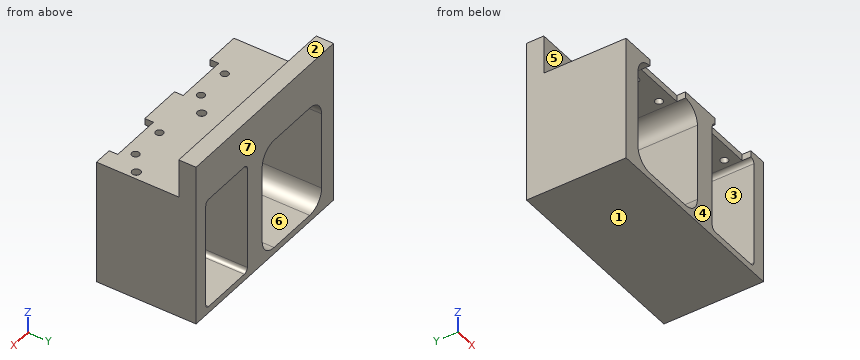
from build123d import *

# Parameters (mm, degrees)
SKETCH1_W                  = 405
SKETCH1_H                  = 295
BOSS_EXTRUDE1_DEPTH        = 53
SKETCH3_OUTSIDE_W          = 507.768
SKETCH3_OUTSIDE_H          = 397.768
SKETCH3_OUTSIDE_W_2        = 369
SKETCH3_OUTSIDE_H_2        = 259
CUT_EXTRUDE2_DEPTH         = 45
MINI_BIN_CUTS_DEPTH        = 46
FILLET1_R                  = 8
SKETCH6_W                  = 259
SKETCH6_H                  = 7
CUT_EXTRUDE5_DEPTH         = 418.533531588
SKETCH8_R                  = 1.75
SKETCH8_R_2                = 1.95
HOLES_LIDS_8_9_12_13_DEPTH = 3
SKETCH9_W                  = 113
SKETCH9_H                  = 46
SKETCH9_W_2                = 199.5
CUT_EXTRUDE6_DEPTH         = 362.718467872
SKETCH10_W                 = 219
SKETCH10_H                 = 46
CUT_EXTRUDE7_DEPTH         = 182.993131739
CUT_EXTRUDE8_REACH         = 121.093
SKETCH11_W                 = 24
SKETCH11_H                 = 4


with BuildPart() as part:
    # Sketch1 → Boss-Extrude1 (new body)
    with BuildSketch(Plane(origin=(0, 0, 0), x_dir=(1, 0, 0), z_dir=(0, 1, 0))):
        Rectangle(SKETCH1_W, SKETCH1_H)
    extrude(amount=BOSS_EXTRUDE1_DEPTH)

    # Sketch3 outside → Cut-Extrude2 (cut)
    with BuildSketch(Plane(origin=(0, 0, 0), x_dir=(-1, 0, 0), z_dir=(0, -1, 0))):
        Rectangle(SKETCH3_OUTSIDE_W, SKETCH3_OUTSIDE_H)
        Rectangle(SKETCH3_OUTSIDE_W_2, SKETCH3_OUTSIDE_H_2, mode=Mode.SUBTRACT)
    extrude(amount=-CUT_EXTRUDE2_DEPTH, mode=Mode.SUBTRACT)

    # Sketch2 → Mini bin cuts (cut)
    with BuildSketch(Plane(origin=(0, 53, 0), x_dir=(1, 0, 0), z_dir=(0, 1, 0))):
        with BuildLine():
            Line((-173.5, -126.5), (-105.5, -126.5))
            ThreePointArc((-105.5, -126.5), (-99.843145751, -124.156854249), (-97.5, -118.5))
            Line((-97.5, -118.5), (-97.5, -49.5))
            ThreePointArc((-97.5, -49.5), (-99.843145751, -43.843145751), (-105.5, -41.5))
            Line((-105.5, -41.5), (-173.5, -41.5))
            ThreePointArc((-173.5, -41.5), (-179.156854249, -43.843145751), (-181.5, -49.5))
            Line((-181.5, -49.5), (-181.5, -118.5))
            ThreePointArc((-181.5, -118.5), (-179.156854249, -124.156854249), (-173.5, -126.5))
        make_face()
        with BuildLine():
            Line((-173.5, -31.5), (-105.5, -31.5))
            ThreePointArc((-105.5, -31.5), (-99.843145751, -29.156854249), (-97.5, -23.5))
            Line((-97.5, -23.5), (-97.5, 40.5))
            ThreePointArc((-97.5, 40.5), (-99.843145751, 46.156854249), (-105.5, 48.5))
            Line((-105.5, 48.5), (-173.5, 48.5))
            ThreePointArc((-173.5, 48.5), (-179.156854249, 46.156854249), (-181.5, 40.5))
            Line((-181.5, 40.5), (-181.5, -23.5))
            ThreePointArc((-181.5, -23.5), (-179.156854249, -29.156854249), (-173.5, -31.5))
        make_face()
        with BuildLine():
            Line((-173.5, 126.5), (-105.5, 126.5))
            ThreePointArc((-105.5, 126.5), (-99.843145751, 124.156854249), (-97.5, 118.5))
            Line((-97.5, 118.5), (-97.5, 66.5))
            ThreePointArc((-97.5, 66.5), (-99.843145751, 60.843145751), (-105.5, 58.5))
            Line((-105.5, 58.5), (-173.5, 58.5))
            ThreePointArc((-173.5, 58.5), (-179.156854249, 60.843145751), (-181.5, 66.5))
            Line((-181.5, 66.5), (-181.5, 118.5))
            ThreePointArc((-181.5, 118.5), (-179.156854249, 124.156854249), (-173.5, 126.5))
        make_face()
        with BuildLine():
            Line((173.5, -126.5), (115.5, -126.5))
            ThreePointArc((115.5, -126.5), (109.843145751, -124.156854249), (107.5, -118.5))
            Line((107.5, -118.5), (107.5, 7.5))
            ThreePointArc((107.5, 7.5), (109.843145751, 13.156854249), (115.5, 15.5))
            Line((115.5, 15.5), (173.5, 15.5))
            ThreePointArc((173.5, 15.5), (179.156854249, 13.156854249), (181.5, 7.5))
            Line((181.5, 7.5), (181.5, -118.5))
            ThreePointArc((181.5, -118.5), (179.156854249, -124.156854249), (173.5, -126.5))
        make_face()
        with BuildLine():
            Line((173.5, 126.5), (107.5, 126.5))
            ThreePointArc((107.5, 126.5), (101.843145751, 124.156854249), (99.5, 118.5))
            Line((99.5, 118.5), (99.5, 33.5))
            ThreePointArc((99.5, 33.5), (101.843145751, 27.843145751), (107.5, 25.5))
            Line((107.5, 25.5), (173.5, 25.5))
            ThreePointArc((173.5, 25.5), (179.156854249, 27.843145751), (181.5, 33.5))
            Line((181.5, 33.5), (181.5, 118.5))
            ThreePointArc((181.5, 118.5), (179.156854249, 124.156854249), (173.5, 126.5))
        make_face()
        with BuildLine():
            Line((81.5, 126.5), (20.5, 126.5))
            ThreePointArc((20.5, 126.5), (14.843145751, 124.156854249), (12.5, 118.5))
            Line((12.5, 118.5), (12.5, -7.5))
            ThreePointArc((12.5, -7.5), (14.843145751, -13.156854249), (20.5, -15.5))
            Line((20.5, -15.5), (81.5, -15.5))
            ThreePointArc((81.5, -15.5), (87.156854249, -13.156854249), (89.5, -7.5))
            Line((89.5, -7.5), (89.5, 118.5))
            ThreePointArc((89.5, 118.5), (87.156854249, 124.156854249), (81.5, 126.5))
        make_face()
        with BuildLine():
            Line((-9.5, 126.5), (-31.5, 126.5))
            ThreePointArc((-31.5, 126.5), (-37.156854249, 124.156854249), (-39.5, 118.5))
            Line((-39.5, 118.5), (-39.5, 11.5))
            ThreePointArc((-39.5, 11.5), (-37.156854249, 5.843145751), (-31.5, 3.5))
            Line((-31.5, 3.5), (-9.5, 3.5))
            ThreePointArc((-9.5, 3.5), (-3.843145751, 5.843145751), (-1.5, 11.5))
            Line((-1.5, 11.5), (-1.5, 118.5))
            ThreePointArc((-1.5, 118.5), (-3.843145751, 124.156854249), (-9.5, 126.5))
        make_face()
        with BuildLine():
            Line((-57.5, 126.5), (-79.5, 126.5))
            ThreePointArc((-79.5, 126.5), (-85.156854249, 124.156854249), (-87.5, 118.5))
            Line((-87.5, 118.5), (-87.5, 11.5))
            ThreePointArc((-87.5, 11.5), (-85.156854249, 5.843145751), (-79.5, 3.5))
            Line((-79.5, 3.5), (-57.5, 3.5))
            ThreePointArc((-57.5, 3.5), (-51.843145751, 5.843145751), (-49.5, 11.5))
            Line((-49.5, 11.5), (-49.5, 118.5))
            ThreePointArc((-49.5, 118.5), (-51.843145751, 124.156854249), (-57.5, 126.5))
        make_face()
        with BuildLine():
            Line((-79.5, -15.5), (-55.5, -15.5))
            ThreePointArc((-55.5, -15.5), (-54.085786438, -16.085786438), (-53.5, -17.5))
            Line((-53.5, -17.5), (-53.5, -65.5))
            ThreePointArc((-53.5, -65.5), (-54.085786438, -66.914213562), (-55.5, -67.5))
            Line((-55.5, -67.5), (-79.5, -67.5))
            ThreePointArc((-79.5, -67.5), (-80.914213562, -66.914213562), (-81.5, -65.5))
            Line((-81.5, -65.5), (-81.5, -17.5))
            ThreePointArc((-81.5, -17.5), (-80.914213562, -16.085786438), (-79.5, -15.5))
        make_face()
        with BuildLine():
            Line((-73.5, -126.5), (-49.5, -126.5))
            ThreePointArc((-49.5, -126.5), (-43.843145751, -124.156854249), (-41.5, -118.5))
            Line((-41.5, -118.5), (-41.5, -82.5))
            ThreePointArc((-41.5, -82.5), (-43.843145751, -76.843145751), (-49.5, -74.5))
            Line((-49.5, -74.5), (-73.5, -74.5))
            ThreePointArc((-73.5, -74.5), (-79.156854249, -76.843145751), (-81.5, -82.5))
            Line((-81.5, -82.5), (-81.5, -118.5))
            ThreePointArc((-81.5, -118.5), (-79.156854249, -124.156854249), (-73.5, -126.5))
        make_face()
        with BuildLine():
            Line((-35.5, -15.5), (-11.5, -15.5))
            ThreePointArc((-11.5, -15.5), (-5.843145751, -17.843145751), (-3.5, -23.5))
            Line((-3.5, -23.5), (-3.5, -59.5))
            ThreePointArc((-3.5, -59.5), (-5.843145751, -65.156854249), (-11.5, -67.5))
            Line((-11.5, -67.5), (-35.5, -67.5))
            ThreePointArc((-35.5, -67.5), (-41.156854249, -65.156854249), (-43.5, -59.5))
            Line((-43.5, -59.5), (-43.5, -23.5))
            ThreePointArc((-43.5, -23.5), (-41.156854249, -17.843145751), (-35.5, -15.5))
        make_face()
        with BuildLine():
            Line((-29.5, -74.5), (-5.5, -74.5))
            ThreePointArc((-5.5, -74.5), (-4.085786438, -75.085786438), (-3.5, -76.5))
            Line((-3.5, -76.5), (-3.5, -124.5))
            ThreePointArc((-3.5, -124.5), (-4.085786438, -125.914213562), (-5.5, -126.5))
            Line((-5.5, -126.5), (-29.5, -126.5))
            ThreePointArc((-29.5, -126.5), (-30.914213562, -125.914213562), (-31.5, -124.5))
            Line((-31.5, -124.5), (-31.5, -76.5))
            ThreePointArc((-31.5, -76.5), (-30.914213562, -75.085786438), (-29.5, -74.5))
        make_face()
        with BuildLine():
            Line((89.5, -126.5), (19.5, -126.5))
            ThreePointArc((19.5, -126.5), (13.843145751, -124.156854249), (11.5, -118.5))
            Line((11.5, -118.5), (11.5, -33.5))
            ThreePointArc((11.5, -33.5), (13.843145751, -27.843145751), (19.5, -25.5))
            Line((19.5, -25.5), (89.5, -25.5))
            ThreePointArc((89.5, -25.5), (95.156854249, -27.843145751), (97.5, -33.5))
            Line((97.5, -33.5), (97.5, -118.5))
            ThreePointArc((97.5, -118.5), (95.156854249, -124.156854249), (89.5, -126.5))
        make_face()
    extrude(amount=-MINI_BIN_CUTS_DEPTH, mode=Mode.SUBTRACT)

    # Fillet1
    fillet1_edges = [part.edges().sort_by_distance(p)[0] for p in [
        (184.5, 22.5, 129.5),
        (184.5, 22.5, -129.5),
        (-184.5, 22.5, -129.5),
        (-184.5, 22.5, 129.5),
    ]]
    fillet(fillet1_edges, radius=FILLET1_R)

    # Sketch6 → Cut-Extrude5 (cut, through all)
    with BuildSketch(Plane.ZY.offset(184.5)):
        with Locations((0, 3.5)):
            Rectangle(SKETCH6_W, SKETCH6_H)
    extrude(amount=-CUT_EXTRUDE5_DEPTH, mode=Mode.SUBTRACT)

    # Sketch8 → Holes Lids 8,9,12,13 (cut)
    with BuildSketch(Plane.XY.offset(129.5)):
        with Locations((-69.5, 16.5)):
            Circle(SKETCH8_R)
        with Locations((-25.5, 16.5)):
            Circle(SKETCH8_R)
        with Locations((46.5, 16.5)):
            Circle(SKETCH8_R)
        with Locations((136.5, 16.5)):
            Circle(SKETCH8_R)
        with Locations((152.5, 16.5)):
            Circle(SKETCH8_R)
        with Locations((62.5, 16.5)):
            Circle(SKETCH8_R)
        with Locations((-9.5, 16.5)):
            Circle(SKETCH8_R)
        with Locations((-53.5, 16.5)):
            Circle(SKETCH8_R)
        with Locations((-44.5, 23)):
            Circle(SKETCH8_R_2)
        with Locations((-0.5, 23)):
            Circle(SKETCH8_R_2)
        with Locations((71.5, 23)):
            Circle(SKETCH8_R_2)
        with Locations((161.5, 23)):
            Circle(SKETCH8_R_2)
    extrude(amount=-HOLES_LIDS_8_9_12_13_DEPTH, mode=Mode.SUBTRACT)

    # Sketch9 → Cut-Extrude6 (cut, through all)
    with BuildSketch(Plane.XY.offset(147.5)):
        with Locations((-146, 30)):
            Rectangle(SKETCH9_W, SKETCH9_H)
        with Locations((102.75, 30)):
            Rectangle(SKETCH9_W_2, SKETCH9_H)
    extrude(amount=-CUT_EXTRUDE6_DEPTH, mode=Mode.SUBTRACT)

    # Sketch10 → Cut-Extrude7 (cut, through all)
    with BuildSketch(Plane(origin=(3, 0, 0), x_dir=(0, 0, -1), z_dir=(1, 0, 0))):
        with Locations((38, 30)):
            Rectangle(SKETCH10_W, SKETCH10_H)
    extrude(amount=-CUT_EXTRUDE7_DEPTH, mode=Mode.SUBTRACT)

    # Cut-Extrude8: up to this face of the body (flat: up to its plane)
    cut_extrude8_end = Plane(part.part.faces().sort_by_distance((-61.5, 30.239473231, 126.5))[0])
    # Sketch11 → Cut-Extrude8 (cut, up to the picked face)
    with BuildSketch(Plane.XY.offset(129.5), mode=Mode.PRIVATE) as cut_extrude8_sk1:
        with Locations((-61.5, 9)):
            Rectangle(SKETCH11_W, SKETCH11_H)
    cut_extrude8_tool1 = split(extrude(cut_extrude8_sk1.sketch, amount=-CUT_EXTRUDE8_REACH, mode=Mode.PRIVATE), bisect_by=cut_extrude8_end, keep=Keep.BOTH, mode=Mode.PRIVATE)
    # Sketch11 → Cut-Extrude8 (cut, up to the picked face)
    with BuildSketch(Plane.XY.offset(129.5), mode=Mode.PRIVATE) as cut_extrude8_sk2:
        with Locations((-17.5, 9)):
            Rectangle(SKETCH11_W, SKETCH11_H)
    cut_extrude8_tool2 = split(extrude(cut_extrude8_sk2.sketch, amount=-CUT_EXTRUDE8_REACH, mode=Mode.PRIVATE), bisect_by=cut_extrude8_end, keep=Keep.BOTH, mode=Mode.PRIVATE)
    add(cut_extrude8_tool1.solids().sort_by(Axis((-61.5, 9, 129.5), (0, 0, -1)))[0], mode=Mode.SUBTRACT)
    add(cut_extrude8_tool2.solids().sort_by(Axis((-17.5, 9, 129.5), (0, 0, -1)))[0], mode=Mode.SUBTRACT)


solid = part.part
Geometry: final body of the model. Coordinates: model frame, mm. Face numbers are marked on the shaded views. A direction names the side the tool comes from. Give positions to 0.01 mm unless a question says otherwise; leave off trailing zeros. Order: outer loops, then holes, each group sorted by start corner. A loop starts at its lowest first (then second) coordinate and runs counter-clockwise, first axis right, second up. Notation, with made-up numbers: (9.25, 68.5) - (28.25, 68.5) arc R29 cw to (28.25, 96.5) - close; hole circle Ø3 at (48, 86). An arc over 180 degrees is marked (long way). Use CSV: the item, a comma, the result in double quotes.
1. Section query B-B (y = 36). Output: boundary loops of the cut face in (x, z).
Answers below:
outline,"(-89.5, 71.5) - (3, 71.5) - (3, 129.5) - (-89.5, 129.5) - close; hole (-81.5, 82.5) arc R8 ccw to (-73.5, 74.5) - (-49.5, 74.5) arc R8 ccw to (-41.5, 82.5) - (-41.5, 118.5) arc R8 ccw to (-49.5, 126.5) - (-73.5, 126.5) arc R8 ccw to (-81.5, 118.5) - close; hole (-31.5, 76.5) arc R2 ccw to (-29.5, 74.5) - (-5.5, 74.5) arc R2 ccw to (-3.5, 76.5) - (-3.5, 124.5) arc R2 ccw to (-5.5, 126.5) - (-29.5, 126.5) arc R2 ccw to (-31.5, 124.5) - close"
2. Section query C-C (x = -17.5). Output: boundary loops of the cut face in (y, z).
Answers below:
outline,"(7, 71.5) - (53, 71.5) - (53, 74.5) - (7, 74.5) - close; (11, 126.5) - (53, 126.5) - (53, 147.5) - (45, 147.5) - (45, 129.5) - (11, 129.5) - close"
3. Contact query for flat-ended pins moving along their axis: pin 1 (0.9 mm diameter, centred on x = -20.5, z = 127.5, fed in from -Y); pin 2 (1.9 mm diameter, centred on x = 0, y = 22, fed in from +Z); pin 3 (5.5 mm diameter, centred on x = -64, z = 142.5, fed in from -Y). Output: stop coordinate, or through.
Answers below:
pin 1,"y = 11"
pin 2,"z = 129.5"
pin 3,"y = 45"
4. Mould query, pull axis Z, two halves, no side actions, for the marked faces 1, 2, 3 and 4. Classes: +Z half, -Z half, draft (parallel to the pull), parting line (faces both ways), or undercut.
Answers below:
face 1,"-Z half"
face 2,"+Z half"
face 3,"undercut"
face 4,"draft"
5. Material intervals for line 1 along X through (y, z) = (40, 90); line 2 along Z through (x, y) = (-58.5, 23.5); line 3 along Z through (x, y) = (-60.5, 49), sorted ascending. Write a range as from..to.
Answers below:
line 1,"-89.5..-81.5, -41.5..-31.5, -3.5..3"
line 2,"71.5..74.5, 126.5..129.5"
line 3,"71.5..74.5, 126.5..147.5"
6. Section query D-D (x = -0.5). Output: boundary loops of the cut face in (y, z), plus the area to 3 significant figures.
Answers below:
outline,"(7, 71.5) - (53, 71.5) - (53, 147.5) - (45, 147.5) - (45, 129.5) - (24.95, 129.5) - (24.95, 126.5) - (21.05, 126.5) - (21.05, 129.5) - (7, 129.5) - close"
area,"2,800 mm2"
7. Section query A-A (z = 92.5). Output: boundary loops of the cut face in (x, y), plus the area to 3 significant figures.
Answers below:
outline,"(-89.5, 7) - (-81.5, 7) - (-81.5, 53) - (-89.5, 53) - close; (-41.5, 7) - (-31.5, 7) - (-31.5, 53) - (-41.5, 53) - close; (-3.5, 7) - (3, 7) - (3, 53) - (-3.5, 53) - close"
area,"1,130 mm2"
8. Access query for the marked faces 5, 6 and 7. Directions: +Z, -Z, +X, -X, +Y, -Y. A direction counts if a zero-diameter tool reaches every point of the face in a straight line with its end or side. Return the directions, or none.
Answers below:
face 5,"+Z, +X, -X, -Y"
face 6,"+Y, -Y"
face 7,"+Z, -Z, +X, -X, +Y"
